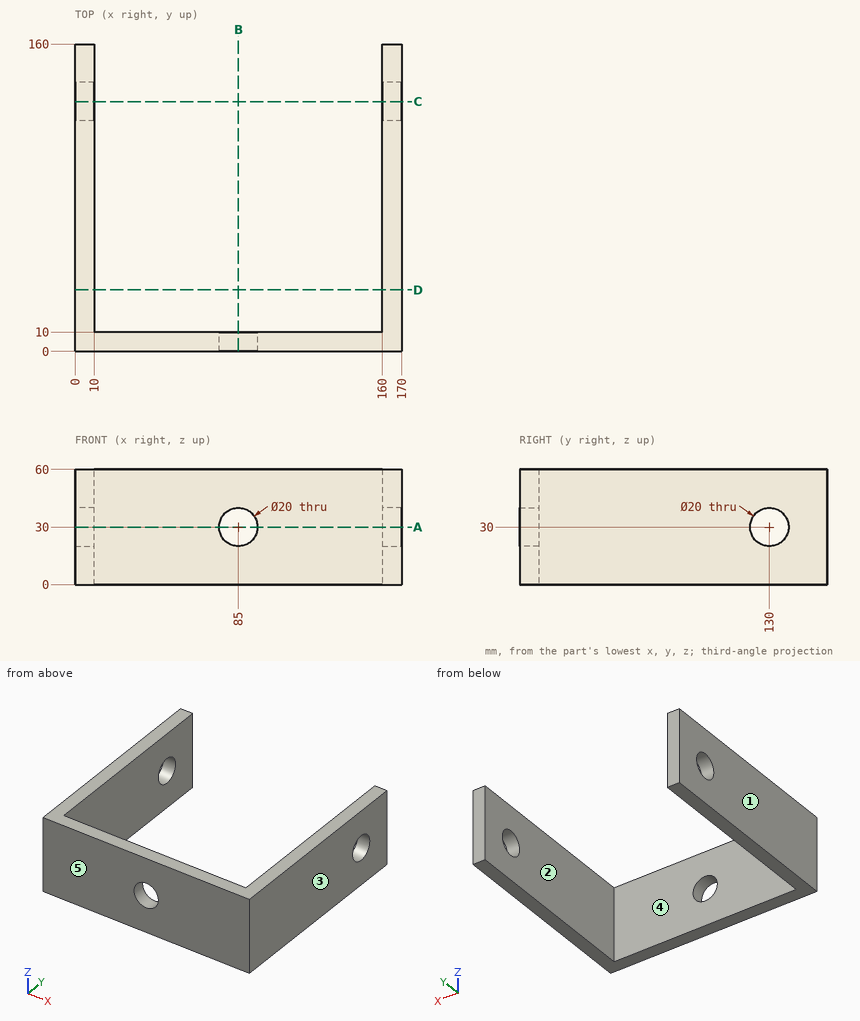
Can you work these out from the drawing? Everything is in mm from the part's minimum corner. A direction names the side the tool comes from. Give positions to 0.01 mm unless a question says otherwise; leave off trailing zeros. Order: outer loops, then holes, each group sorted by start corner. A loop starts at its lowest first (then second) coordinate and runs counter-clockwise, first axis right, second up. Notation, with made-up numbers: M -38.5,-13.5 L -19.5,-13.5 A30 ccw -19.5,10.5 Z; hole C 22,-27 d11. An arc over 180 degrees is marked long. Use a Markdown table: item, result. Add a question column.
Item 1: Suppose I cut it at B-B (x = 85). List the corners of the cut face in (y, z) for me, then the cut area to 3 significant figures.
Item 2: We'd pull the mould along X, two halves only. Please class the marked faces 1, 2 and 3: +X half, -X half, draft (parallel to the pull), parting line (faces both ways), or undercut.
Item 3: Suppose I cut it at D-D (y = 32). List the corners of the cut face in (x, z) for me, then the cut area to 3 significant figures.
Item 4: Suppose I cut it at A-A (z = 30). List the corners of the cut face in (x, y) for me, then the cut area to 3 significant figures.
Item 5: If I drill on L1, parallel to Y at x = 5.25, z = 30; L2, parallel to X at y = 128, z = 45; L3, parallel to Z at x = 85, y = 6.25, over which ranges is the centre line in solid material (lowest first)? Write a range as [from, to].
Item 6: Will this pin go through, and if not, where does the flat tip stop? pin 1 (3 mm diameter, centred on x = 58.5, z = 47.5, fed in from +Y).
Item 7: Suppose I cut it at C-C (y = 130). List the corners of the cut face in (x, z) for me, then the cut area to 3 significant figures.
Item 8: For the marked faces 4 and 5, which set-ups out of +Z, -Z, +X, -X, +Y, -Y let a thin tool reach every point of the face, with its end or its side?
Answer sheet:
| question | item | result |
|---|---|---|
| 1 | outline | M 0,0 L 10,0 L 10,20 L 0,20 Z; M 0,40 L 10,40 L 10,60 L 0,60 Z |
| 1 | area | 400 mm² |
| 2 | face 1 | -X half |
| 2 | face 2 | undercut |
| 2 | face 3 | +X half |
| 3 | outline | M 0,0 L 10,0 L 10,60 L 0,60 Z; M 160,0 L 170,0 L 170,60 L 160,60 Z |
| 3 | area | 1,200 mm² |
| 4 | outline | M 0,0 L 75,0 L 75,10 L 10,10 L 10,120 L 0,120 Z; M 0,140 L 10,140 L 10,160 L 0,160 Z; M 95,0 L 170,0 L 170,120 L 160,120 L 160,10 L 95,10 Z; M 160,140 L 170,140 L 170,160 L 160,160 Z |
| 4 | area | 4,100 mm² |
| 5 | L1 | y = [0, 120], [140, 160] |
| 5 | L2 | x = [0, 10], [160, 170] |
| 5 | L3 | z = [0, 20], [40, 60] |
| 6 | pin 1 | stops at y = 10 |
| 7 | outline | M 0,0 L 10,0 L 10,20 L 0,20 Z; M 0,40 L 10,40 L 10,60 L 0,60 Z; M 160,0 L 170,0 L 170,20 L 160,20 Z; M 160,40 L 170,40 L 170,60 L 160,60 Z |
| 7 | area | 800 mm² |
| 8 | face 4 | +Z, -Z, +Y |
| 8 | face 5 | +Z, -Z, +X, -X, -Y |
